Autodesk Fusion 360 part; units mm, degrees
sketch "Sketch1" plane through (0, 0, 0) normal (0, 0, 1) x (1, 0, 0)
  line L0 (0, 0) -> (170, 0)
  line L1 (170, 0) -> (170, 70)
  line L2 (170, 70) -> (0, 70)
  line L3 (0, 70) -> (0, 0)
  line L4 (0, 70) -> (10, 70)
  line L5 (10, 70) -> (10, 0)
  line L6 (10, 0) -> (0, 0)
  line L7 (0, 0) -> (0, 70)
  line L8 (0, 10) -> (170, 10)
  line L9 (170, 10) -> (170, 0)
  line L10 (170, 0) -> (0, 0)
  line L11 (0, 0) -> (0, 10)
  line L12 (170, 0) -> (160, 0)
  line L13 (160, 0) -> (160, 70)
  line L14 (160, 70) -> (170, 70)
  line L15 (170, 70) -> (170, 0)
  dimension "d1" = 170
  dimension "d2" = 70
extrude "Extrude1" add sketch "Sketch1" along normal blind 2 contours L2 L5 L8 L13
extrude "Extrude2" add sketch "Sketch1" along normal blind 60 contours L0 L3 L5 L6 L7 L8 L10 L11 | L0 L5 L8 L10 L13 | L2 L3 L4 L5 L7 L8 | L0 L1 L8 L9 L10 L12 L13 L15 | L1 L2 L8 L13 L14 L15
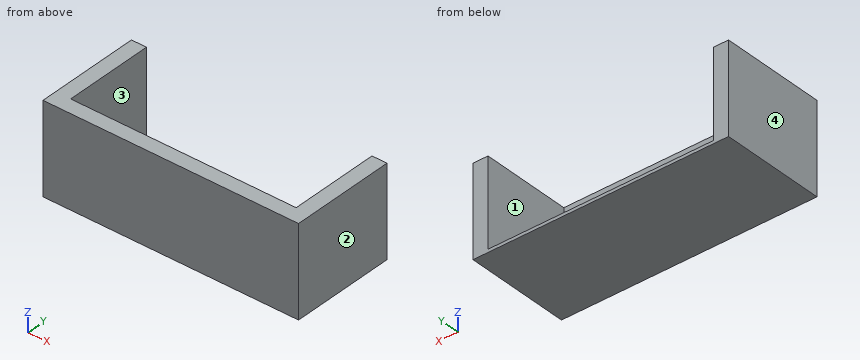
Input: part model. Units: mm. Frame: model coordinates. Face numbers are marked on the shaded views. Round coordinates to 2 decimals unless told otherwise and drop trailing zeros. Write each loop counter-clockwise with the first axis right and the second up, starting at its lowest first coordinate (ties: lowest second). Pieces come first, ordered by that corner, then holes.
1) Cut plane B-B (y = 55). Return the cut outline in (x, z).
2) Cut plane C-C (x = 86). Return the cut outline in (y, z).
3) Contact query for flat-ended pins moving along their axis: P1, Ø2, axis at x = 132.5, y = 56, coming from the +Z side; P2, Ø6, axis at x = 116.5, z = 17, coming from the +Y side. Output: stop coordinate, or through.
4) Cut plane A-A (z = 6.5). Return the cut outline in (x, y), then the cut area to 3 significant figures.
5) Ray query, L1, parallel to X at y = 64.5, z = 4.5; L2, parallel to Y at x = 113.5, z = 7; L3, parallel to Z at x = 70, y = 61. Return the intervals inside material, ascending.
6) Draft query along X for the marked faces 1, 2, 3 and 4. Return one class per face: pulls with the +X half, pulls with the -X half, needs draft (parallel to the pull), parting line crosses it, or undercut.
Geometry says:
1. outline: (0, 0) - (170, 0) - (170, 60) - (160, 60) - (160, 2) - (10, 2) - (10, 60) - (0, 60) - close
2. outline: (0, 0) - (70, 0) - (70, 2) - (10, 2) - (10, 60) - (0, 60) - close
3. P1: stops at z = 2
3. P2: stops at y = 10
4. outline: (0, 0) - (170, 0) - (170, 70) - (160, 70) - (160, 10) - (10, 10) - (10, 70) - (0, 70) - close
4. area: 2,900 mm2
5. L1: x = 0 to 10, 160 to 170
5. L2: y = 0 to 10
5. L3: z = 0 to 2
6. face 1: undercut
6. face 2: pulls with the +X half
6. face 3: undercut
6. face 4: pulls with the -X half
